Verification items for the finished model (mm, model axes). A direction names the side the tool comes from. Round coordinates to 2 decimals unless told otherwise and drop trailing zeros. Order: outer loops, then holes, each group sorted by start corner. A loop starts at its lowest first (then second) coordinate and runs counter-clockwise, first axis right, second up. Notation, with made-up numbers: (3.5, 39.5) -> (39.5, 39.5) arc R22 cw to (39.5, 62.5) -> close; hole circle Ø2 at (44.5, 33). An arc over 180 degrees is marked (long way). Put each result on its own line as item: value.
```python
from build123d import *

# Parameters (mm, degrees)
F0_R     = 2
F1_DEPTH = 110


with BuildPart() as f1:
    # F0 (on Front) → F1 (new body)
    with BuildSketch(Plane.XZ):
        with BuildLine():
            ThreePointArc((15, 13.5), (14.56066, 14.56066), (13.5, 15))
            Line((13.5, 15), (4, 15))
            ThreePointArc((4, 15), (3.292893, 14.707107), (3, 14))
            Line((3, 14), (3, 13))
            ThreePointArc((3, 13), (3.292893, 12.292893), (4, 12))
            Line((4, 12), (7.464466, 12))
            ThreePointArc((7.464466, 12), (8.388346, 11.382683), (8.171573, 10.292893))
            Line((8.171573, 10.292893), (3.318019, 5.43934))
            ThreePointArc((3.318019, 5.43934), (2.831384, 5.114181), (2.257359, 5))
            Line((2.257359, 5), (-2.257359, 5))
            ThreePointArc((-2.257359, 5), (-2.831384, 5.114181), (-3.318019, 5.43934))
            Line((-3.318019, 5.43934), (-8.171573, 10.292893))
            ThreePointArc((-8.171573, 10.292893), (-8.388346, 11.382683), (-7.464466, 12))
            Line((-7.464466, 12), (-4, 12))
            ThreePointArc((-4, 12), (-3.292893, 12.292893), (-3, 13))
            Line((-3, 13), (-3, 14))
            ThreePointArc((-3, 14), (-3.292893, 14.707107), (-4, 15))
            Line((-4, 15), (-13.5, 15))
            ThreePointArc((-13.5, 15), (-14.56066, 14.56066), (-15, 13.5))
            Line((-15, 13.5), (-15, 4))
            ThreePointArc((-15, 4), (-14.707107, 3.292893), (-14, 3))
            Line((-14, 3), (-13, 3))
            ThreePointArc((-13, 3), (-12.292893, 3.292893), (-12, 4))
            Line((-12, 4), (-12, 7.464466))
            ThreePointArc((-12, 7.464466), (-11.382683, 8.388346), (-10.292893, 8.171573))
            Line((-10.292893, 8.171573), (-5, 2.87868))
            Line((-5, 2.87868), (-5, -2.257359))
            ThreePointArc((-5, -2.257359), (-5.114181, -2.831384), (-5.43934, -3.318019))
            Line((-5.43934, -3.318019), (-10.292893, -8.171573))
            ThreePointArc((-10.292893, -8.171573), (-11.382683, -8.388346), (-12, -7.464466))
            Line((-12, -7.464466), (-12, -4))
            ThreePointArc((-12, -4), (-12.292893, -3.292893), (-13, -3))
            Line((-13, -3), (-14, -3))
            ThreePointArc((-14, -3), (-14.707107, -3.292893), (-15, -4))
            Line((-15, -4), (-15, -13.5))
            ThreePointArc((-15, -13.5), (-14.56066, -14.56066), (-13.5, -15))
            Line((-13.5, -15), (-4, -15))
            ThreePointArc((-4, -15), (-3.292893, -14.707107), (-3, -14))
            Line((-3, -14), (-3, -13))
            ThreePointArc((-3, -13), (-3.292893, -12.292893), (-4, -12))
            Line((-4, -12), (-7.464466, -12))
            ThreePointArc((-7.464466, -12), (-8.388346, -11.382683), (-8.171573, -10.292893))
            Line((-8.171573, -10.292893), (-3.318019, -5.43934))
            ThreePointArc((-3.318019, -5.43934), (-2.831384, -5.114181), (-2.257359, -5))
            Line((-2.257359, -5), (2.257359, -5))
            ThreePointArc((2.257359, -5), (2.831384, -5.114181), (3.318019, -5.43934))
            Line((3.318019, -5.43934), (8.171573, -10.292893))
            ThreePointArc((8.171573, -10.292893), (8.388346, -11.382683), (7.464466, -12))
            Line((7.464466, -12), (4, -12))
            ThreePointArc((4, -12), (3.292893, -12.292893), (3, -13))
            Line((3, -13), (3, -14))
            ThreePointArc((3, -14), (3.292893, -14.707107), (4, -15))
            Line((4, -15), (13.5, -15))
            ThreePointArc((13.5, -15), (14.56066, -14.56066), (15, -13.5))
            Line((15, -13.5), (15, -4))
            ThreePointArc((15, -4), (14.707107, -3.292893), (14, -3))
            Line((14, -3), (13, -3))
            ThreePointArc((13, -3), (12.292893, -3.292893), (12, -4))
            Line((12, -4), (12, -7.464466))
            ThreePointArc((12, -7.464466), (11.382683, -8.388346), (10.292893, -8.171573))
            Line((10.292893, -8.171573), (5.43934, -3.318019))
            ThreePointArc((5.43934, -3.318019), (5.114181, -2.831384), (5, -2.257359))
            Line((5, -2.257359), (5, 2.257359))
            ThreePointArc((5, 2.257359), (5.114181, 2.831384), (5.43934, 3.318019))
            Line((5.43934, 3.318019), (10.292893, 8.171573))
            ThreePointArc((10.292893, 8.171573), (11.382683, 8.388346), (12, 7.464466))
            Line((12, 7.464466), (12, 4))
            ThreePointArc((12, 4), (12.292893, 3.292893), (13, 3))
            Line((13, 3), (14, 3))
            ThreePointArc((14, 3), (14.707107, 3.292893), (15, 4))
            Line((15, 4), (15, 13.5))
        make_face()
        Circle(F0_R, mode=Mode.SUBTRACT)
    extrude(amount=-F1_DEPTH)


solid = f1.part
```
Item 1: Sectioned sample at B-B, the plane z = 0. Record the boundary of the cut face in (x, y).
Geometry check:
outline: (-5, 0) -> (-2, 0) -> (-2, 110) -> (-5, 110) -> close; (2, 0) -> (5, 0) -> (5, 110) -> (2, 110) -> close
Item 2: Depth check by flat-ended pin: pin 1 Ø3 at (x, z) = (7.5, 2) entering from -Y; pin 2 Ø1.4 at (x, y) = (0.5, 62.5) entering from +Z; pin 3 Ø1.5 at (y, z) = (54, 1) entering from -X; pin 4 Ø1 at (y, z) = (84, 1.5) entering from +X. Enter the tip coordinate at first touch or a pass-through.
Geometry check:
pin 1: through
pin 2: z = 5
pin 3: x = -5
pin 4: x = 5
Item 3: Release check for a two-part mould opening along X. For faces 1 (the face through (-15, 54, 9)), 2 (the face through (5, 54, 0)), 3 (the face through (-5.71, 54.23, 7.83)) record: pulls with the +X half, pulls with the -X half, needs draft (parallel to the pull), parting line crosses it, or undercut.
Geometry check:
face 1: pulls with the -X half
face 2: pulls with the +X half
face 3: undercut
Item 4: Sectioned sample at A-A, the plane x = 0. Record the boundary of the cut face in (y, z), then the cut area to 3 significant figures.
Geometry check:
outline: (0, -5) -> (110, -5) -> (110, -2) -> (0, -2) -> close; (0, 2) -> (110, 2) -> (110, 5) -> (0, 5) -> close
area: 660 mm2
Item 5: Tool access check on faces 4 (the face through (-5.78, 54.23, -7.9)), 5 (the face through (9, 54, -15)), 6 (the face through (0, 54, 5)), 7 (the face through (-5, 54, 0)). Record the directions out of +Z, -Z, +X, -X, +Y, -Y that give a thin tool (end or side, any length) a straight path to the whole face; none if there is none.
Geometry check:
face 4: +Y, -Y
face 5: -Z, +X, -X, +Y, -Y
face 6: +Z, +Y, -Y
face 7: -X, +Y, -Y
Item 6: Material ranges on line 1 along Z through (x, y) = (0, 26); line 2 along X through (y, z) = (27.5, 7); line 3 along Z through (x, y) = (-5.5, 49), recorded low to high.
Geometry check:
line 1: -5 to -2, 2 to 5
line 2: -15 to -12, -9.12 to -4.88, 4.88 to 9.12, 12 to 15
line 3: -15 to -12, -7.62 to -3.38, 3.38 to 7.62, 12 to 15
